from build123d import *

# Parameters (mm, degrees)
F0_W     = 105.7792007923
F0_H     = 79.7204598784
F0_W_2   = 90.3369858861
F0_H_2   = 65.0503486395
F1_DEPTH = 67.564
F2_W     = 43.8358001411
F2_H     = 33.7584646449
F3_DEPTH = 96.012
F4_R     = 9.6723299626
F5_DEPTH = 129.032


with BuildPart() as f1:
    # F0 (on Top) → F1 (new body)
    with BuildSketch(Plane.XY):
        Rectangle(F0_W, F0_H)
        Rectangle(F0_W_2, F0_H_2, mode=Mode.SUBTRACT)
    extrude(amount=F1_DEPTH)

    # F2 (on face) → F3 (cut)
    with BuildSketch(Plane.XZ.offset(39.8602299392)):
        with Locations((0, 50.6847676775)):
            Rectangle(F2_W, F2_H)
    extrude(amount=-F3_DEPTH, mode=Mode.SUBTRACT)

    # F4 (on face) → F5 (cut)
    with BuildSketch(Plane.YZ.offset(52.8896003962)):
        with Locations((0, 33.4872640669)):
            Circle(F4_R)
    extrude(amount=-F5_DEPTH, mode=Mode.SUBTRACT)


solid = f1.part
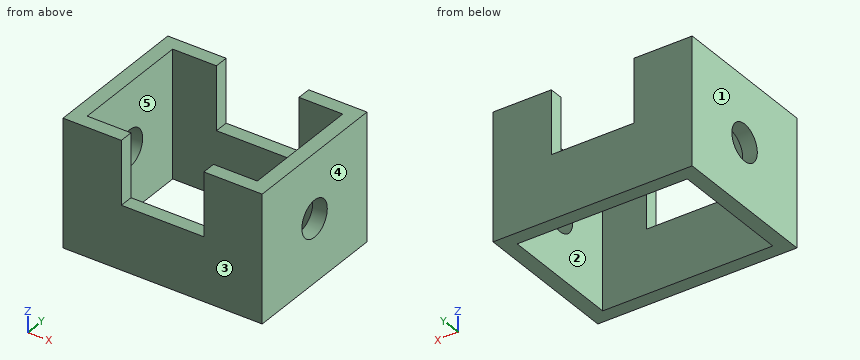
Input: part model. Units: mm. Frame: model coordinates. Face numbers are marked on the shaded views. A direction names the side the tool comes from. Coordinates: 2 decimals unless noted, no trailing zeros. Order: outer loops, then holes, each group sorted by start corner. A loop starts at its lowest first (then second) coordinate and runs counter-clockwise, first axis right, second up.
1. Draft query along X for the marked faces 3, 4 and 5. Return one class per face: +X half, -X half, draft (parallel to the pull), parting line (faces both ways), or undercut.
Checked values:
face 3: draft
face 4: +X half
face 5: undercut
2. Cut plane D-D, the plane y = -30. Return loops of the section in (x, z).
Checked values:
outline: (-52.89, 0) - (-45.17, 0) - (-45.17, 67.56) - (-52.89, 67.56) - close; (45.17, 0) - (52.89, 0) - (52.89, 67.56) - (45.17, 67.56) - close
3. Access query for the marked faces 1 and 2. Directions: +Z, -Z, +X, -X, +Y, -Y. A direction counts if a zero-diameter tool reaches every point of the face in a straight line with its end or side. Return the directions, or none.
Checked values:
face 1: +Z, -Z, -X, +Y, -Y
face 2: +Z, -Z
4. Cut plane A-A, the plane y = 0. Return loops of the section in (x, z), plus the area to 3 significant figures.
Checked values:
outline: (-52.89, 0) - (-45.17, 0) - (-45.17, 23.81) - (-52.89, 23.81) - close; (-52.89, 43.16) - (-45.17, 43.16) - (-45.17, 67.56) - (-52.89, 67.56) - close; (45.17, 0) - (52.89, 0) - (52.89, 23.81) - (45.17, 23.81) - close; (45.17, 43.16) - (52.89, 43.16) - (52.89, 67.56) - (45.17, 67.56) - close
area: 745 mm2
5. Ray query, line 1 along Y through (x, z) = (-10.5, 20); line 2 along Z through (x, y) = (48, 0); line 3 along X through (y, z) = (10.5, 23.5). Return the intervals inside material, ascending.
Checked values:
line 1: y = -39.86 to -32.53, 32.53 to 39.86
line 2: z = 0 to 23.81, 43.16 to 67.56
line 3: x = -52.89 to -45.17, 45.17 to 52.89
6. Cut plane C-C, the plane z = 48. Return loops of the section in (x, y).
Checked values:
outline: (-52.89, -39.86) - (-21.92, -39.86) - (-21.92, -32.53) - (-45.17, -32.53) - (-45.17, 32.53) - (-21.92, 32.53) - (-21.92, 39.86) - (-52.89, 39.86) - close; (21.92, -39.86) - (52.89, -39.86) - (52.89, 39.86) - (21.92, 39.86) - (21.92, 32.53) - (45.17, 32.53) - (45.17, -32.53) - (21.92, -32.53) - close
7. Contact query for a flat-ended pin moving along its axis: P1, Ø8, axis at x = -7, y = 35, coming from the +Z side. Output: stop coordinate, or through.
Checked values:
P1: stops at z = 33.81
8. Cut plane B-B, the plane x = 42.5. Return loops of the section in (y, z).
Checked values:
outline: (-39.86, 0) - (-32.53, 0) - (-32.53, 67.56) - (-39.86, 67.56) - close; (32.53, 0) - (39.86, 0) - (39.86, 67.56) - (32.53, 67.56) - close
